Work out the finished part from the listing and answer in its coordinate system (mm). Face numbers are marked on the shaded views. Give positions to 0.01 mm unless a question says otherwise; leave off trailing zeros. Loops run counter-clockwise (first coordinate to the right, second up) from the corner with the lowest first, then second, coordinate; pieces in that order, holes last. Notation, with made-up numbers: (65, 24.25) -> (76, 24.25) arc R13 ccw to (76, 49.25) -> close; hole circle Ø2 at (-8, 30). An arc over 180 degrees is marked (long way). Answer as CSV lines item,"result". Start each with the question number.
1. Find section A-A, the plane x = -17.5. Give the vertices of the cut face in (y, z), and give its area (3 significant figures).
2. Find section D-D, the plane x = -1. Give the vertices of the cut face in (y, z).
3. Find section C-C, the plane z = -14.5. Give the vertices of the cut face in (x, y).
4. Find the intervals of material crossed by line 1 along Z through (x, y) = (-28.5, 3.5); line 2 along X through (y, z) = (3, 18); line 3 along Y through (x, z) = (29, -19.5), in increasing order.
5. Find section B-B, the plane y = 2.9. Give the vertices of the cut face in (x, z), and give its area (3 significant figures).
6. A flat-ended cylindrical pin translates along its axis: pin 1 Ø1 at (x, z) = (-7.5, -18) entering from +Y. Find the tip coordinate at first contact, or state that the pin passes through.
7. Determine the mould class of the marked faces 1 and 2 for opening direction Z: +Z half, -Z half, draft (parallel to the pull), parting line (faces both ways), or undercut.
Autodesk Inventor part; units mm, degrees
ref_plane "YZ Plane" through (0, 0, 0) normal (1, 0, 0) x (0, 1, 0)
ref_plane "XZ Plane" through (0, 0, 0) normal (0, 1, 0) x (-1, 0, 0)
ref_plane "XY Plane" through (0, 0, 0) normal (0, 0, 1) x (1, 0, 0)
sketch "Boceto1" plane through (0, 0, 0) normal (0, 1, 0) x (-1, 0, 0)
  line L0 (-38, -25) -> (38, -25)
  line L1 (38, -25) -> (38, 25)
  line L2 (38, 25) -> (-38, 25)
  line L3 (-38, 25) -> (-38, -25)
  line L4 (-38, -25) -> (38, 25) construction
  line L5 (38, -25) -> (-38, 25) construction
  point P0 (0, 0)
  dimension "d0" = 76
  dimension "d1" = 50
extrude "Extrusión1" add sketch "Boceto1" along normal blind 2
sketch "Boceto2" plane through (0, 2, 0) normal (0, 1, 0) x (1, 0, 0)
  line L0 (38, 25) -> (-38, 25)
  line L1 (-38, -25) -> (-10, -25)
  line L2 (-38, -25) -> (38, -25)
  line L3 (-38, -25) -> (-38, 25)
  line L4 (-38, 25) -> (-10, 25)
  line L5 (-10, 23) -> (-36, 23)
  line L6 (-36, 23) -> (-36, -23)
  line L7 (-36, -23) -> (-10, -23)
  line L8 (-10, 25) -> (-10, 23)
  line L9 (-10, -23) -> (-10, -25)
  point P0 (0, 0)
  point P1 (0, 25)
  dimension "d14" = 2
extrude "Extrusión4" add sketch "Boceto2" along normal blind 2
sketch "Boceto5" plane through (-38, 0, 25) normal (0, 0, 1) x (1, 0, 0)
  line L0 (28, 2) -> (28, 4)
  line L1 (28, 4) -> (28, 2)
  line L2 (76, 2) -> (28, 2)
  line L3 (28, 2) -> (30, 4)
  line L4 (28, 2) -> (32.2548, 2) construction
  line L5 (28, 4) -> (30, 4)
  point P0 (38, 0)
extrude "Extrusión5" add sketch "Boceto5" against normal blind 2
mirror "Simetría2" about plane through (0, 0, 0) normal (0, 0, 1) of "Extrusión5"
properties part number "Mirror"
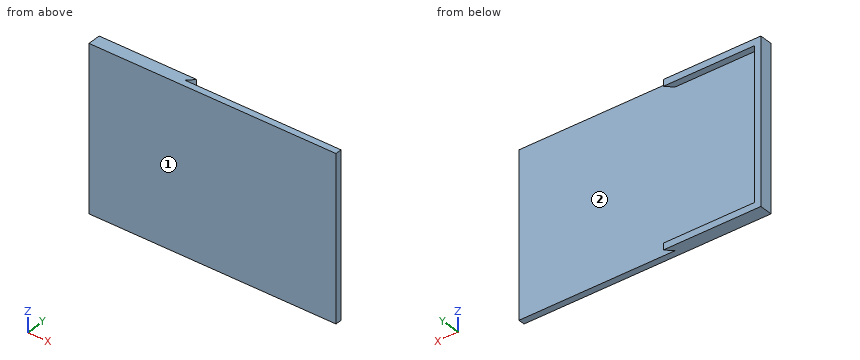
Resolved:
1,outline,"(0, -25) -> (4, -25) -> (4, -23) -> (2, -23) -> (2, 23) -> (4, 23) -> (4, 25) -> (0, 25) -> close"
1,area,"108 mm^2"
2,outline,"(0, -25) -> (2, -25) -> (2, 25) -> (0, 25) -> close"
3,outline,"(-38, 0) -> (38, 0) -> (38, 2) -> (-36, 2) -> (-36, 4) -> (-38, 4) -> close"
4,line 1,"z = -25 to -23, 23 to 25"
4,line 2,"x = -38 to -36"
4,line 3,"y = 0 to 2"
5,outline,"(-38, -25) -> (-9.1, -25) -> (-9.1, -23) -> (-36, -23) -> (-36, 23) -> (-9.1, 23) -> (-9.1, 25) -> (-38, 25) -> close"
5,area,"208 mm^2"
6,pin 1,"stops at y = 2"
7,face 1,"draft"
7,face 2,"undercut"
